Study the drawing (mm; zero at the part's minimum x, y, z) and answer. Round coordinates to 2 decimals unless told otherwise and drop trailing zeros. Write each loop counter-clockwise with the first axis right and the second up, starting at its lowest first coordinate (ties: lowest second). Pieces come first, ordered by that corner, then holes. Notation, with made-up numbers: M 21,39 L 26,39 A20 ccw 26,63 Z; hole C 39,-20.75 d4. An arc over 180 degrees is marked long. Write each question's results on one line, items separated by ' | '.
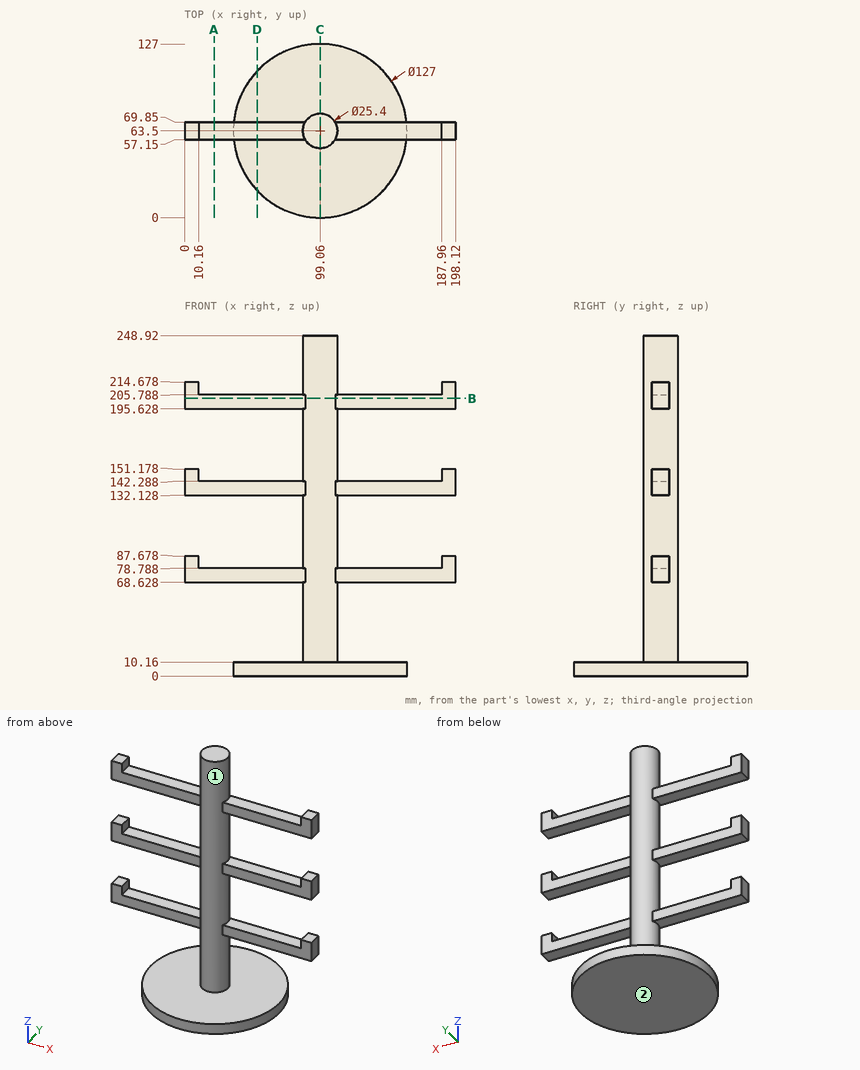
1) Section B-B (z = 203) is taken. Determine the outline of the cut face in (x, y), then the cut area to 3 significant figures.
Return value:
outline: M 0,57.15 L 88.06,57.15 A12.7 ccw 110.06,57.15 L 198.12,57.15 L 198.12,69.85 L 110.06,69.85 A12.7 ccw 88.06,69.85 L 0,69.85 Z | area: 2,710 mm²
2) Section D-D (x = 53) is taken. Determine the outline of the cut face in (y, z), then the cut area to 3 significant figures.
Return value:
outline: M 19.79,0 L 107.21,0 L 107.21,10.16 L 19.79,10.16 Z; M 57.15,68.63 L 69.85,68.63 L 69.85,78.79 L 57.15,78.79 Z; M 57.15,132.13 L 69.85,132.13 L 69.85,142.29 L 57.15,142.29 Z; M 57.15,195.63 L 69.85,195.63 L 69.85,205.79 L 57.15,205.79 Z | area: 1,280 mm²
3) The mould has two halves that part along Z. Classify the marked faces 1 and 2: +Z half, -Z half, draft (parallel to the pull), parting line (faces both ways), or undercut.
Return value:
face 1: undercut | face 2: -Z half
4) Section C-C (x = 99.06) is taken. Determine the outline of the cut face in (y, z).
Return value:
outline: M 0,0 L 127,0 L 127,10.16 L 76.2,10.16 L 76.2,248.92 L 50.8,248.92 L 50.8,10.16 L 0,10.16 Z
5) Each of these flat-tipped pins is pushed along its axis until it touches: pin 1 (12 mm diameter, centred on x = 71, z = 136.5, fed in from +Y); pin 2 (15 mm diameter, centred on x = 23, z = 142.5, fed in from -Y); pin 3 (2 mm diameter, centred on y = 75.5, z = 132.5, fed in from -X); pin 4 (8 mm diameter, centred on y = 46.5, z = 80, fed in from +X). Where does it stop, or does it pass through?
Return value:
pin 1: y = 69.85 | pin 2: y = 57.15 | pin 3: x = 92.71 | pin 4: through
6) Section A-A (x = 21.5) is taken. Determine the outline of the cut face in (y, z).
Return value:
outline: M 57.15,68.63 L 69.85,68.63 L 69.85,78.79 L 57.15,78.79 Z; M 57.15,132.13 L 69.85,132.13 L 69.85,142.29 L 57.15,142.29 Z; M 57.15,195.63 L 69.85,195.63 L 69.85,205.79 L 57.15,205.79 Z
7) Find the intervals of material crossed by line 1 (Z direction, x = 142, y = 58); line 2 (Z direction, x = 100.5, y = 103); line 3 (Y direction, x = 102, z = 220) (1 decimal), in increasing order.
Return value:
line 1: 0 to 10.16, 68.63 to 78.79, 132.13 to 142.29, 195.63 to 205.79 | line 2: 0 to 10.16 | line 3: 51.1 to 75.9
